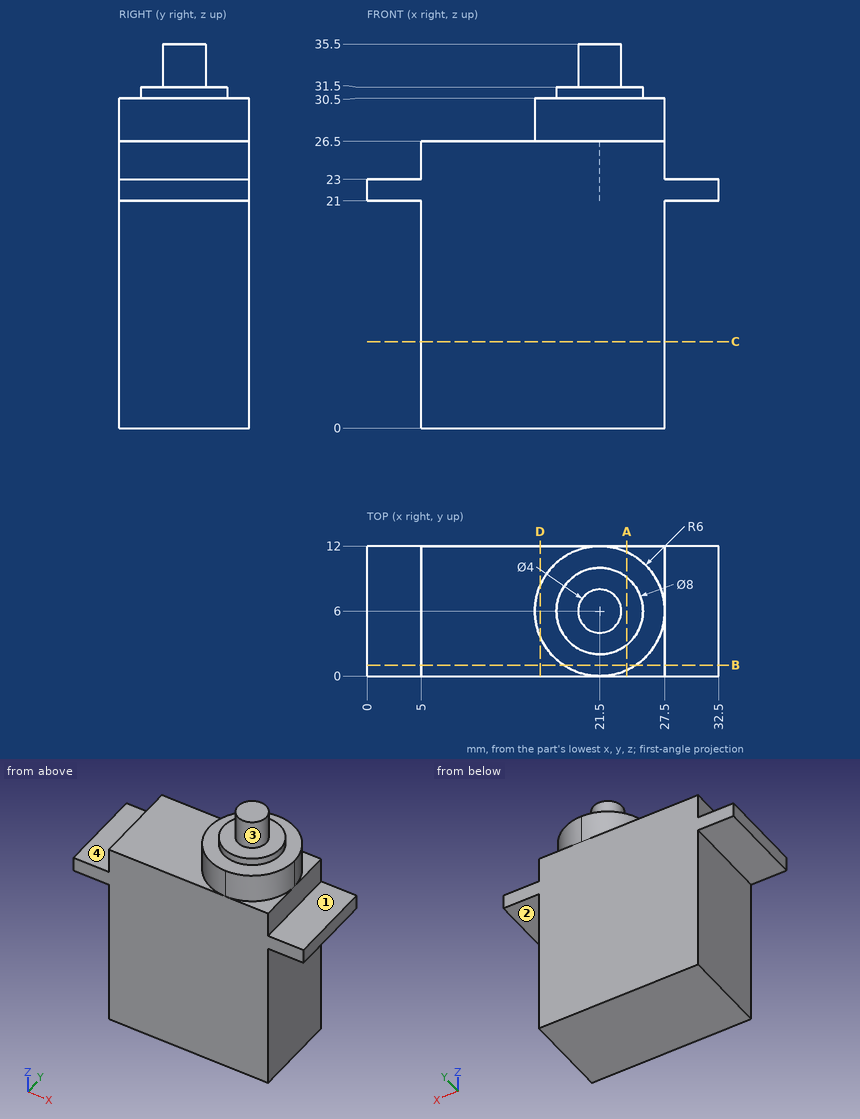
Geometry check sheet. Reference: drawing and pictorial views, mm from the part's lowest x, y, z. A direction names the side the tool comes from. Give positions to 0.01 mm unless a question says otherwise; leave off trailing zeros. Order: outer loops, then holes, each group sorted by start corner. A loop starts at its lowest first (then second) coordinate and runs counter-clockwise, first axis right, second up. Notation, with made-up numbers: M 41,-24 L 63,-24 A20 cw 63,-17 Z; hole C 63.5,72 d9. An arc over 180 degrees is marked long. Answer as a JSON object with one key per item and string values. Group by question number.
1) Cross-section at A-A (x = 24). Enter the section's corners in (y, z), then the cut area to 3 significant figures.
2) Cross-section at C-C (z = 8). Enter the section's corners in (x, y), then the cut area to 3 significant figures.
3) Cross-section at B-B (y = 1). Enter the section's corners in (x, z), then the cut area to 3 significant figures.
4) Depth check by flat-ended pin: pin 1 Ø3 at (y, z) = (2.5, 10.5) entering from -X; pin 2 Ø4 at (x, y) = (30.5, 5.5) entering from -Z; pin 3 Ø3.5 at (x, y) = (12, 6) entering from +Z. Enter the tip coordinate at first touch or a pass-through.
5) Cross-section at D-D (x = 16). Enter the section's corners in (y, z).
6) Scan lines: line 1 along Z through (x, y) = (8.5, 10.25); line 2 along Z through (x, y) = (18, 7.5); line 3 along X through (y, z) = (10.75, 14). Record each from-to range of solid material in increasing order. Write a range as [from, to].
7) Access from +Z, -Z, +X, -X, +Y, -Y to the whole of each face (thin tool, end or side, straight path). Record for the marked faces 1, 2, 3 and 4.
Result sheet:
{
 "1": {"outline": "M 0,0 L 12,0 L 12,26.5 L 11.45,26.5 L 11.45,30.5 L 9.12,30.5 L 9.12,31.5 L 2.88,31.5 L 2.88,30.5 L 0.55,30.5 L 0.55,26.5 L 0,26.5 Z", "area": "368 mm2"},
 "2": {"outline": "M 5,0 L 27.5,0 L 27.5,12 L 5,12 Z", "area": "270 mm2"},
 "3": {"outline": "M 0,21 L 5,21 L 5,0 L 27.5,0 L 27.5,21 L 32.5,21 L 32.5,23 L 27.5,23 L 27.5,26.5 L 24.82,26.5 L 24.82,30.5 L 18.18,30.5 L 18.18,26.5 L 5,26.5 L 5,23 L 0,23 Z", "area": "643 mm2"},
 "4": {"pin 1": "stops at x = 5", "pin 2": "stops at z = 21", "pin 3": "stops at z = 26.5"},
 "5": {"outline": "M 0,0 L 12,0 L 12,26.5 L 8.4,26.5 L 8.4,30.5 L 3.6,30.5 L 3.6,26.5 L 0,26.5 Z"},
 "6": {"line 1": "z = [0, 26.5]", "line 2": "z = [0, 31.5]", "line 3": "x = [5, 27.5]"},
 "7": {"face 1": "+Z, +X, +Y, -Y", "face 2": "-Z, +X, +Y, -Y", "face 3": "+Z", "face 4": "+Z, -X, +Y, -Y"}
}
